Input: dimensioned drawing with shaded views. Units: mm. Origin: part minimum x, y, z. A direction names the side the tool comes from. Give positions to 0.01 mm unless a question says otherwise; leave off trailing zeros. Loops run counter-clockwise (first coordinate to the right, second up) from the corner with the lowest first, then second, coordinate; pieces in that order, holes last.
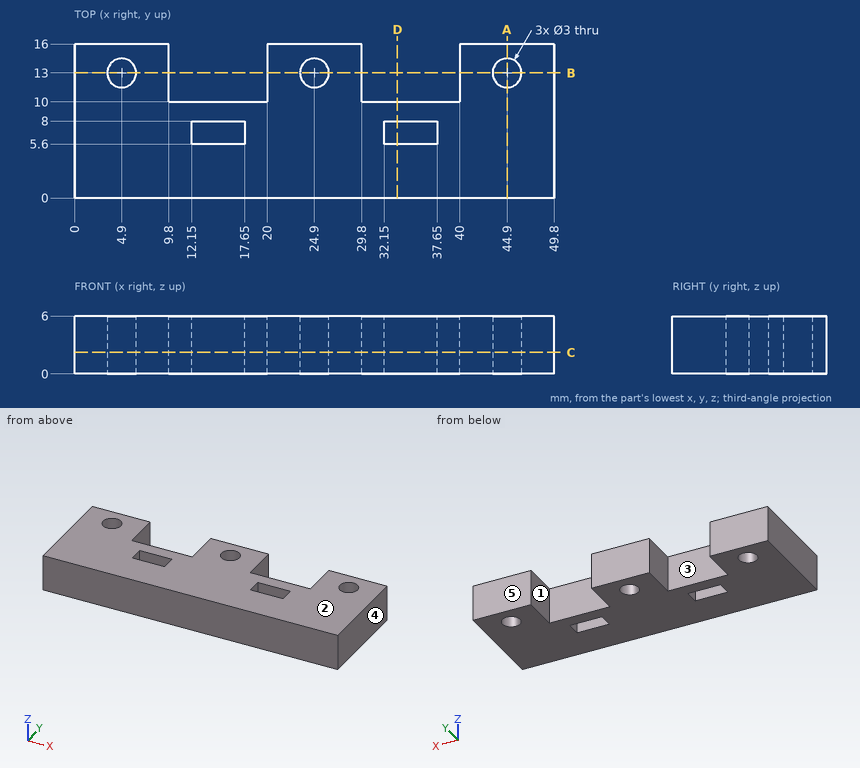
(1) Reachability of the marked faces 1 and 2 from +Z, -Z, +X, -X, +Y, -Y: full face, straight path, thin tool, end or side. Return the list, or none.
A:
face 1: +Z, -Z, +Y
face 2: +Z, +X, -X, +Y, -Y
(2) Section A-A, the plane x = 44.9. Return the cut outline in (y, z).
A:
outline: (0, 0) - (11.5, 0) - (11.5, 6) - (0, 6) - close; (14.5, 0) - (16, 0) - (16, 6) - (14.5, 6) - close
(3) Section B-B, the plane y = 13. Return the cut outline in (x, z).
A:
outline: (0, 0) - (3.4, 0) - (3.4, 6) - (0, 6) - close; (6.4, 0) - (9.8, 0) - (9.8, 6) - (6.4, 6) - close; (20, 0) - (23.4, 0) - (23.4, 6) - (20, 6) - close; (26.4, 0) - (29.8, 0) - (29.8, 6) - (26.4, 6) - close; (40, 0) - (43.4, 0) - (43.4, 6) - (40, 6) - close; (46.4, 0) - (49.8, 0) - (49.8, 6) - (46.4, 6) - close
(4) Ray query, line 1 along X through (y, z) = (15, 1.6); line 2 along X through (y, z) = (5.75, 4.5); line 3 along Y through (x, z) = (37, 3.4). Return the intervals inside material, ascending.
A:
line 1: x = 0 to 9.8, 20 to 29.8, 40 to 49.8
line 2: x = 0 to 12.15, 17.65 to 32.15, 37.65 to 49.8
line 3: y = 0 to 5.6, 8 to 10
(5) Section C-C, the plane z = 2.25. Return the cut outline in (x, y).
A:
outline: (0, 0) - (49.8, 0) - (49.8, 16) - (40, 16) - (40, 10) - (29.8, 10) - (29.8, 16) - (20, 16) - (20, 10) - (9.8, 10) - (9.8, 16) - (0, 16) - close; hole circle Ø3 at (4.9, 13); hole (12.15, 5.6) - (17.65, 5.6) - (17.65, 8) - (12.15, 8) - close; hole circle Ø3 at (24.9, 13); hole (32.15, 5.6) - (37.65, 5.6) - (37.65, 8) - (32.15, 8) - close; hole circle Ø3 at (44.9, 13)
(6) Mould query, pull axis X, two halves, no side actions, for the marked faces 3, 4 and 5. Classes: pulls with the +X half, pulls with the -X half, needs draft (parallel to the pull), parting line crosses it, or undercut.
A:
face 3: undercut
face 4: pulls with the +X half
face 5: needs draft
(7) Section D-D, the plane x = 33.5. Return the cut outline in (y, z), then the cut area to 3 significant figures.
A:
outline: (0, 0) - (5.6, 0) - (5.6, 6) - (0, 6) - close; (8, 0) - (10, 0) - (10, 6) - (8, 6) - close
area: 45.6 mm2
(8) First-contact query: pin 1 (2.5 mm diameter, centred on x = 16, z = 2, fed in from +Y). Flat tip, straight axial feed; report the tip coordinate or a pass-through.
A:
pin 1: stops at y = 10
